Geometry: final body of the model. Coordinates: model frame, mm. A direction names the side the tool comes from. Round coordinates to 2 decimals unless told otherwise and drop trailing zeros. Write each loop counter-clockwise with the first axis right and the second up, starting at its lowest first coordinate (ties: lowest second). Pieces come first, ordered by that corner, then holes.
from build123d import *

# Parameters (mm, degrees)
F0_W     = 16
F0_H     = 36
F1_DEPTH = 5
F3_DEPTH = 12
F4_R     = 2
F5_R     = 5


with BuildPart() as f1:
    # F0 (on Top) → F1 (new body)
    with BuildSketch(Plane.XY):
        with Locations((0, 10)):
            Rectangle(F0_W, F0_H)
        with BuildLine():
            ThreePointArc((-4, 20), (0, 24), (4, 20))
            Line((4, 20), (4, 0))
            ThreePointArc((4, 0), (0, -4), (-4, 0))
            Line((-4, 0), (-4, 20))
        make_face(mode=Mode.SUBTRACT)
    extrude(amount=F1_DEPTH)

    # F2 (on Top) → F3 (join)
    with BuildSketch(Plane.XY):
        Polygon((18, -8), (0, -8), (-18, -8), (-18, -14), (18, -14), align=None)
    extrude(amount=F3_DEPTH)

    # F4
    f4_edges = [f1.edges().sort_by_distance(p)[0] for p in [
        (-18, -14, 6),
        (-18, -8, 6),
        (18, -8, 6),
        (18, -14, 6),
        (0, -8, 5),
        (8, -8, 2.5),
        (-8, -8, 2.5),
    ]]
    fillet(f4_edges, radius=F4_R)

    # F5
    f5_edges = [f1.edges().sort_by_distance(p)[0] for p in [
        (-8, 28, 2.5),
        (8, 28, 2.5),
    ]]
    fillet(f5_edges, radius=F5_R)


solid = f1.part
1) Line query: probe 1 along X at (y, z) = (12, 3.25); probe 2 along X at (y, z) = (-5.5, 3.25); probe 3 along X at (y, z) = (-1, 1.5). Output: solid intervals per line, ascending.
2) Section D-D on z = 9.5. Output: boundary loops of the cut face in (x, y).
3) Draft query along Y for faces 1 (the cylindrical face through (7, 26, 3)), 2 (the flat face through (-18, -11, 6)), 3 (the cylindrical face through (0, 24, 2)). Return one class per face: pulls with the +Y half, pulls with the -Y half, needs draft (parallel to the pull), parting line crosses it, or undercut.
4) Section C-C on z = 3.5. Output: boundary loops of the cut face in (x, y), plus the area to 3 significant figures.
5) Section B-B on x = 0. Output: boundary loops of the cut face in (y, z), plus the area to 3 significant figures.
6) Reachability of faces 4 (the flat face through (-4, 10, 2)), 5 (the flat face through (8, 8, 2)), 6 (the flat face through (0.2, -8, 7.2)) from +Z, -Z, +X, -X, +Y, -Y: full face, straight path, thin tool, end or side. Return the list, or none.
7) Section A-A on y = 9.5. Output: boundary loops of the cut face in (x, z).
8) First-contact query: P1, Ø5, axis at x = -3.5, y = 9, coming from the +Z side; P2, Ø1.5, axis at y = 5.5, z = 2, coming from the +X side; P3, Ø4, axis at x = -10.5, z = 6, coming from the +Y side. Flat tips, straight axial feed; report the tip coordinate or a pass-through.
Filled in:
1. probe 1: x = -8 to -4, 4 to 8
1. probe 2: x = -8 to 8
1. probe 3: x = -8 to -3.87, 3.87 to 8
2. outline: (-18, -12) arc R2 ccw to (-16, -14) - (16, -14) arc R2 ccw to (18, -12) - (18, -10) arc R2 ccw to (16, -8) - (-16, -8) arc R2 ccw to (-18, -10) - close
3. face 1: pulls with the +Y half
3. face 2: needs draft
3. face 3: undercut
4. outline: (-18, -12) arc R2 ccw to (-16, -14) - (16, -14) arc R2 ccw to (18, -12) - (18, -10) arc R2 ccw to (16, -8) - (10, -8) arc R2 cw to (8, -6) - (8, 23) arc R5 ccw to (3, 28) - (-3, 28) arc R5 ccw to (-8, 23) - (-8, -6) arc R2 cw to (-10, -8) - (-16, -8) arc R2 ccw to (-18, -10) - close; hole (-4, 0) arc R4 ccw to (4, 0) - (4, 20) arc R4 ccw to (-4, 20) - close
4. area: 569 mm2
5. outline: (-14, 0) - (-4, 0) - (-4, 5) - (-6, 5) arc R2 cw to (-8, 7) - (-8, 12) - (-14, 12) - close; (24, 0) - (28, 0) - (28, 5) - (24, 5) - close
5. area: 113 mm2
6. face 4: +Z, -Z
6. face 5: +Z, -Z, +X, +Y
6. face 6: +Z, +Y
7. outline: (-8, 0) - (-4, 0) - (-4, 5) - (-8, 5) - close; (4, 0) - (8, 0) - (8, 5) - (4, 5) - close
8. P1: stops at z = 5
8. P2: stops at x = 8
8. P3: stops at y = -7.38
